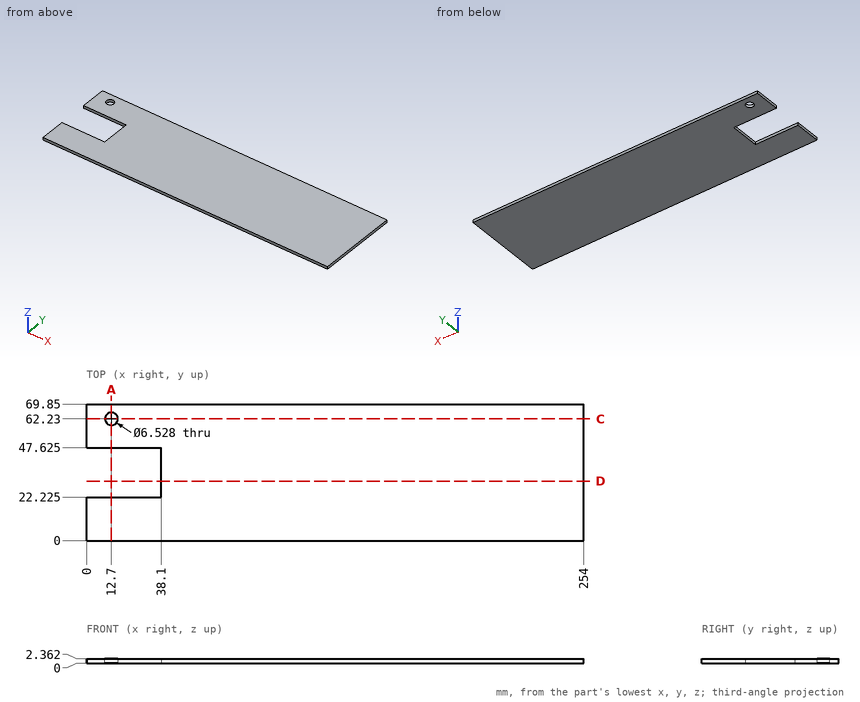
Design review of the part shown in the three views and the two pictorial views. Dimensions are in mm from the part's minimum x, y and z. Round coordinates to 2 decimals unless told otherwise and drop trailing zeros. Order: outer loops, then holes, each group sorted by start corner. A loop starts at its lowest first (then second) coordinate and runs counter-clockwise, first axis right, second up.
Item 1: For pin 1 (1.2 mm diameter, centred on y = 34.5, z = 1, fed in from -X), flat-tipped, find the tip position at first contact; note if it passes through.
Working result:
pin 1: stops at x = 38.1
Item 2: To check wall thickness, follow probe 1 along X at (y, z) = (42, 0.5). State the ranges of the line that lie inside material, in increasing order.
Working result:
probe 1: x = 38.1 to 254
Item 3: Add section A-A, the plane x = 12.7. Count the separate pieces of the cut face and the enclosed holes in it.
Working result:
separate pieces: 3
enclosed holes: 0
Item 4: Add section D-D, the plane y = 30.5. State the section outline as (x, z) points, and give its area (3 significant figures).
Working result:
outline: (38.1, 0) - (254, 0) - (254, 2.36) - (38.1, 2.36) - close
area: 510 mm2
Item 5: Add section C-C, the plane y = 62.23. State the section outline as (x, z) points.
Working result:
outline: (0, 0) - (9.44, 0) - (9.44, 2.36) - (0, 2.36) - close; (15.96, 0) - (254, 0) - (254, 2.36) - (15.96, 2.36) - close
